Part model, mm, in its own coordinate system. Face numbers are marked on the shaded views. A direction names the side the tool comes from. Give positions to 0.01 mm unless a question says otherwise; leave off trailing zeros. Order: outer loops, then holes, each group sorted by start corner. A loop starts at its lowest first (then second) coordinate and runs counter-clockwise, first axis right, second up. Notation, with made-up numbers: (11, 75.25) -> (66, 75.25) arc R38 cw to (66, 113.25) -> close; hole circle Ø7 at (3, -38.5). An arc over 180 degrees is marked (long way). Write item = value, one per line. Start each with the question number.
(1) Probe line 1 along X through (y, z) = (163, -30); line 2 along Z through (x, y) = (114, 182.5). List the from-to ranges inside material, lowest first. Write a range as from..to.
(2) Flat gauge pin, fed straight in: pin 1 (11 mm diameter, centred on x = -29, z = 71, fed in from -Y). Where does the tip first touch, or does it go through?
(3) Saw through at D-D, the plane x = 165. List the corners of the cut face in (y, z).
(4) Which spindle directions (+Z, -Z, +X, -X, +Y, -Y) get a long thin tool onto all of the face, cutting with end or side? Do the marked faces 1 and 2. Say none if no direction does.
(5) Saw through at C-C, the plane y = 132. List the corners of the cut face in (x, z), then the cut area to 3 significant figures.
(6) Saw through at A-A, the plane y = 17. List the corners of the cut face in (x, z), then the cut area to 3 significant figures.
(7) Saw through at B-B, the plane z = -7. List the corners of the cut face in (x, y).
(8) Two-plate mould, pull along X, no slides. Class the marked faces 3, 4 and 5: pulls with the +X half, pulls with the -X half, needs draft (parallel to the pull), parting line crosses it, or undercut.
from build123d import *

# Parameters (mm, degrees)
SKETCH1_W           = 400
SKETCH1_H           = 150
BOSS_EXTRUDE1_DEPTH = 200
SKETCH2_W           = 380
SKETCH2_H           = 130
CUT_EXTRUDE1_DEPTH  = 200
SKETCH3_W           = 200
SKETCH3_H           = 120
CUT_EXTRUDE2_DEPTH  = 20
SKETCH4_W           = 400
SKETCH4_H           = 200
CUT_EXTRUDE3_DEPTH  = 10


with BuildPart() as part:
    # Sketch1 → Boss-Extrude1 (new body)
    with BuildSketch(Plane(origin=(0, 0, 0), x_dir=(1, 0, 0), z_dir=(0, 1, 0))):
        Rectangle(SKETCH1_W, SKETCH1_H)
    extrude(amount=BOSS_EXTRUDE1_DEPTH)

    # Sketch2 → Cut-Extrude1 (cut)
    with BuildSketch(Plane(origin=(0, 200, 0), x_dir=(1, 0, 0), z_dir=(0, 1, 0))):
        Rectangle(SKETCH2_W, SKETCH2_H)
    extrude(amount=-CUT_EXTRUDE1_DEPTH, mode=Mode.SUBTRACT)

    # Sketch3 → Cut-Extrude2 (cut)
    with BuildSketch(Plane.XY.offset(75)):
        with Locations((0, 60)):
            Rectangle(SKETCH3_W, SKETCH3_H)
    extrude(amount=-CUT_EXTRUDE2_DEPTH, mode=Mode.SUBTRACT)

    # Sketch4 → Cut-Extrude3 (cut)
    with BuildSketch(Plane(origin=(0, 0, -75), x_dir=(-1, 0, 0), z_dir=(0, 0, -1))):
        with Locations((0, 100)):
            Rectangle(SKETCH4_W, SKETCH4_H)
    extrude(amount=-CUT_EXTRUDE3_DEPTH, mode=Mode.SUBTRACT)


solid = part.part
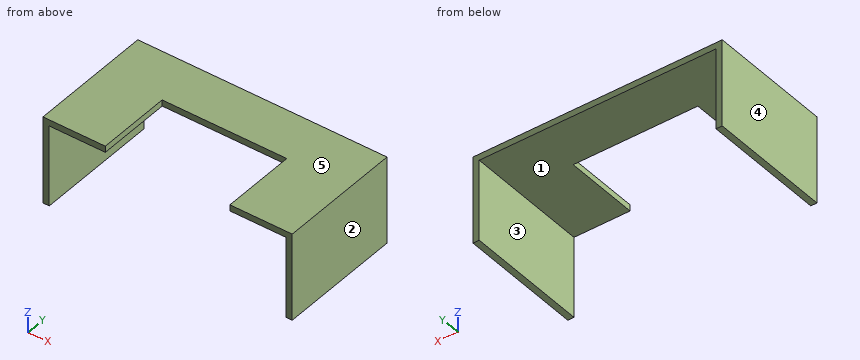
Results list:
q1.line_1 = -200..-190, 190..200
q1.line_2 = 65..75
q2.pin_1 = 120
q3.outline = (0, 65) -> (200, 65) -> (200, 75) -> (0, 75) -> close
q4.face_1 = -Z, +Y, -Y
q4.face_2 = +Z, -Z, +X, +Y, -Y
q5.outline = (-200, -65) -> (-190, -65) -> (-190, 65) -> (190, 65) -> (190, -65) -> (200, -65) -> (200, 75) -> (-200, 75) -> close
q5.area = 6,600 mm^2
q6.outline = (-200, -65) -> (-190, -65) -> (-190, 65) -> (-100, 65) -> (-100, 75) -> (-200, 75) -> close; (100, 65) -> (190, 65) -> (190, -65) -> (200, -65) -> (200, 75) -> (100, 75) -> close
q6.area = 4,600 mm^2
q7.outline = (-200, 0) -> (-190, 0) -> (-190, 200) -> (-200, 200) -> close; (190, 0) -> (200, 0) -> (200, 200) -> (190, 200) -> close
q8.face_3 = undercut
q8.face_4 = pulls with the -X half
q8.face_5 = needs draft
